Verification items for the finished model (mm, model axes). A direction names the side the tool comes from. Coordinates: 2 decimals unless noted, no trailing zeros. Loops run counter-clockwise (first coordinate to the right, second up) from the corner with the lowest first, then second, coordinate; pieces in that order, holes last. Notation, with made-up numbers: (37, 29) -> (87, 29) arc R25 ccw to (87, 56) -> close; hole circle Ø6 at (56.5, 5). An arc over 180 degrees is marked (long way). Answer as a JSON object with one key per item and string values. Group by question number.
Q1. Cross-section at C-C on y = 2.55. Record the boundary of the cut face in (x, z).
Q2. Cross-section at A-A on x = -94.7. Record the boundary of the cut face in (y, z).
Q3. Gauge pin test, flat ends, axial feed: pin 1 Ø2.5 at (x, z) = (-94.7, 91) entering from +Y; pin 2 Ø1.5 at (x, y) = (-96.5, 1) entering from +Z; pin 3 Ø0.9 at (y, z) = (1, 145.5) entering from -X. Record the tip position at first contact, or that the pin passes through.
Q4. Cross-section at B-B on z = 91. Record the boundary of the cut face in (x, y).
Q5. Set-up check for faces 4 (the flat face through (-44, 1, 155)), 5 (the flat face through (-90, 1, 143)): record each of +Z, -Z, +X, -X, +Y, -Y from which the full face is reachable in a straight line by a thin tool's end or side.
Q6. Scan lines: L1, parallel to X at y = 1.4, z = 148.7; L2, parallel to X at y = 2.1, z = 10.2; L3, parallel to X at y = 2.3, z = 91. Record each from-to range of solid material in increasing order.
Q7. Release check for a two-part mould opening along X. For faces 1 (the flat face through (-108.4, 1, 65)), 2 (the flat face through (-100, 1, 128)), 3 (the cylindrical face through (-95.56, 1.52, 93.08)) record: released by +X, released by -X, zero draft, split by the parting line, or undercut.
```python
from build123d import *

# Parameters (mm, degrees)
BOSS_EXTRUDE1_DEPTH = 3
SKETCH2_R           = 2.25
CUT_EXTRUDE1_DEPTH  = 190.168073416
FILLET1_R           = 2


with BuildPart() as part:
    # Sketch1 → Boss-Extrude1 (new body)
    with BuildSketch(Plane(origin=(0, 0, 0), x_dir=(1, 0, 0), z_dir=(0, 1, 0))):
        Polygon((0, 0), (0, -155), (-90, -155), (-90, -128), (-108.4, -128), (-108.4, 0), align=None)
    extrude(amount=BOSS_EXTRUDE1_DEPTH)

    # Sketch2 → Cut-Extrude1 (cut, through all)
    with BuildSketch(Plane(origin=(0, 3, 0), x_dir=(1, 0, 0), z_dir=(0, 1, 0))):
        with Locations(Location((-68.4, -148.7, 0), (0, 0, 270))):
            Circle(SKETCH2_R)
        with Locations(Location((-15.5, -148.7, 0), (0, 0, 270))):
            Circle(SKETCH2_R)
        with Locations(Location((-94.7, -91, 0), (0, 0, 270))):
            Circle(SKETCH2_R)
        with Locations(Location((-61.7, -10.2, 0), (0, 0, 270))):
            Circle(SKETCH2_R)
    extrude(amount=-CUT_EXTRUDE1_DEPTH, mode=Mode.SUBTRACT)

    # Fillet1
    fillet1_edges = [part.edges().sort_by_distance(p)[0] for p in [
        (-90, 1.5, 128),
    ]]
    fillet(fillet1_edges, radius=FILLET1_R)


solid = part.part
```
Computed values:
{
 "1": {"outline": "(-108.4, 0) -> (0, 0) -> (0, 155) -> (-90, 155) -> (-90, 130) arc R2 cw to (-92, 128) -> (-108.4, 128) -> close; hole circle Ø4.5 at (-94.7, 91); hole circle Ø4.5 at (-68.4, 148.7); hole circle Ø4.5 at (-61.7, 10.2); hole circle Ø4.5 at (-15.5, 148.7)"},
 "2": {"outline": "(0, 0) -> (3, 0) -> (3, 88.75) -> (0, 88.75) -> close; (0, 93.25) -> (3, 93.25) -> (3, 128) -> (0, 128) -> close"},
 "3": {"pin 1": "passes through", "pin 2": "stops at z = 128", "pin 3": "stops at x = -90"},
 "4": {"outline": "(-108.4, 0) -> (-96.95, 0) -> (-96.95, 3) -> (-108.4, 3) -> close; (-92.45, 0) -> (0, 0) -> (0, 3) -> (-92.45, 3) -> close"},
 "5": {"face 4": "+Z, +X, -X, +Y, -Y", "face 5": "+Z, -X, +Y, -Y"},
 "6": {"L1": "x = -90 to -70.65, -66.15 to -17.75, -13.25 to 0", "L2": "x = -108.4 to -63.95, -59.45 to 0", "L3": "x = -108.4 to -96.95, -92.45 to 0"},
 "7": {"face 1": "released by -X", "face 2": "zero draft", "face 3": "undercut"}
}
